The listing builds one solid part. Answer for the finished solid, in the listing's coordinates (mm). A direction names the side the tool comes from. Round coordinates to 2 decimals unless told otherwise and drop trailing zeros. Write each loop counter-clockwise with the first axis right and the second up, starting at its lowest first coordinate (ties: lowest second). Pieces come first, ordered by that corner, then holes. Notation, with made-up numbers: (-0.75, 22.25) - (4.25, 22.25) arc R26 cw to (4.25, 49.25) - close; hole circle Ø3 at (4.25, 38.5). An arc over 180 degrees is marked (long way). Answer as CSV lines item,"result". Start each with the question number.
Item 1: A cutting plane is placed at D-D on x = 12. Determine the outline of the cut face in (y, z).
Item 2: A flat-ended cylindrical pin translates along its axis: pin 1 (1.5 mm diameter, centred on y = -6.5, z = 69.5, fed in from -X). Find the tip coordinate at first contact, or state that the pin passes through.
Item 3: Straight lines are drawn through the part: line 1 along Y through (x, z) = (69, 32); line 2 along Y through (x, z) = (19, 39.5); line 3 along Z through (x, y) = (15.5, -20.25) (3 decimals). For each, find the intervals that lie inside material, in ascending order. Write a range as [from, to].
Item 4: A cutting plane is placed at A-A on z = 47. Determine the outline of the cut face in (x, y).
Item 5: Which of the six approach directions +Z, -Z, +X, -X, +Y, -Y give full straight-line access (tool end or side, diameter ignored) to faces 1 (the flat face through (62.255, -20.07, 47.465)), 2 (the flat face through (47.465, -20.07, 62.745)), 3 (the flat face through (39, -15, 41)), 4 (the flat face through (39, -12, 0))?
Item 6: For a pull along X with two mould halves and no side action, classify faces 5 (the flat face through (0, -12, 39)), 6 (the flat face through (17.255, -19.93, 32.465)), 7 (the flat face through (80, -12, 39)), 8 (the flat face through (47.465, -20.07, 17.745)) as pulls with the +X half, pulls with the -X half, needs draft (parallel to the pull), parting line crosses it, or undercut.
Item 7: A cutting plane is placed at B-B on y = -19. Determine the outline of the cut face in (x, z), and give its area (3 significant figures).
Item 8: A cutting plane is placed at C-C on z = 17. Determine the outline of the cut face in (x, y).
```python
from build123d import *

# Parameters (mm, degrees)
F0_W     = 80
F0_H     = 80
F1_DEPTH = 25
F3_DEPTH = 85
F5_DEPTH = 85


with BuildPart() as f1:
    # F0 (on Front) → F1 (new body)
    with BuildSketch(Plane.XZ):
        with Locations((40, 40)):
            Rectangle(F0_W, F0_H)
    extrude(amount=F1_DEPTH)

    # F2 (on face) → F3 (cut)
    with BuildSketch(Plane(origin=(0, 0, 0), x_dir=(0, -1, 0), z_dir=(-1, 0, 0))):
        Polygon((25, 45), (15, 50), (15, 30), (25, 35), (25, 40), align=None)
    extrude(amount=-F3_DEPTH, mode=Mode.SUBTRACT)

    # F4 (on face) → F5 (cut)
    with BuildSketch(Plane.XY.offset(80)):
        Polygon((50, -15), (30, -15), (35, -25), (40, -25), (45, -25), align=None)
    extrude(amount=-F5_DEPTH, mode=Mode.SUBTRACT)


solid = f1.part
```
Geometry says:
1,outline,"(-25, 0) - (0, 0) - (0, 80) - (-25, 80) - (-25, 45) - (-15, 50) - (-15, 30) - (-25, 35) - close"
2,pin 1,"stops at x = 0"
3,line 1,"y = [-25, -19], [-15, 0]"
3,line 2,"y = [-15, 0]"
3,line 3,"z = [0, 32.625], [47.375, 80]"
4,outline,"(0, -25) - (35, -25) - (33, -21) - (0, -21) - close; (0, -15) - (80, -15) - (80, 0) - (0, 0) - close; (45, -25) - (80, -25) - (80, -21) - (47, -21) - close"
5,face 1,"+X, -X"
5,face 2,"+Z, -Z"
5,face 3,"none"
5,face 4,"-Z, +X, -X, +Y, -Y"
6,face 5,"pulls with the -X half"
6,face 6,"needs draft"
6,face 7,"pulls with the +X half"
6,face 8,"undercut"
7,outline,"(0, 0) - (32, 0) - (32, 32) - (0, 32) - close; (0, 48) - (32, 48) - (32, 80) - (0, 80) - close; (48, 0) - (80, 0) - (80, 32) - (48, 32) - close; (48, 48) - (80, 48) - (80, 80) - (48, 80) - close"
7,area,"4,100 mm^2"
8,outline,"(0, -25) - (35, -25) - (30, -15) - (50, -15) - (45, -25) - (80, -25) - (80, 0) - (0, 0) - close"
